from build123d import *

# Parameters (mm, degrees)
BOSS_EXTRUDE1_DEPTH = 25.4
SKETCH2_R           = 6
SKETCH2_R_2         = 5
CUT_EXTRUDE1_DEPTH  = 26.4
FILLET1_R           = 5


with BuildPart() as part:
    # Sketch1 → Boss-Extrude1 (new body)
    with BuildSketch(Plane(origin=(0, 0, 0), x_dir=(0, 0, -1), z_dir=(1, 0, 0))):
        with BuildLine():
            Line((12.7, 0), (12.7, -12.7))
            Line((12.7, -12.7), (38.1, -12.7))
            Line((38.1, -12.7), (38.1, -25.5))
            Line((38.1, -25.5), (-38.1, -25.5))
            Line((-38.1, -25.5), (-38.1, -12.7))
            Line((-38.1, -12.7), (-38.1, 0))
            Line((-38.1, 0), (-12.7, 0))
            ThreePointArc((-12.7, 0), (0, 12.7), (12.7, 0))
        make_face()
    extrude(amount=BOSS_EXTRUDE1_DEPTH)

    # Sketch2 → Cut-Extrude1 (cut, through all)
    with BuildSketch(Plane(origin=(25.4, 0, 0), x_dir=(0, 0, -1), z_dir=(1, 0, 0))):
        Circle(SKETCH2_R)
        with Locations((-25.2, -7.7)):
            Circle(SKETCH2_R_2)
    extrude(amount=-CUT_EXTRUDE1_DEPTH, mode=Mode.SUBTRACT)

    # Fillet1
    fillet1_edges = [part.edges().sort_by_distance(p)[0] for p in [
        (12.7, 0, 38.1),
    ]]
    fillet(fillet1_edges, radius=FILLET1_R)


solid = part.part
Source: CAD feature listing. Evaluate the final solid. Frame: model axes, mm. A direction names the side the tool comes from. Round coordinates to 2 decimals unless told otherwise and drop trailing zeros. Loops run counter-clockwise (first coordinate to the right, second up) from the corner with the lowest first, then second, coordinate; pieces in that order, holes last.
Q1. Mould query, pull axis Y, two halves, no side actions, for faces 4 (the face through (13, -25.5, -1)), 5 (the face through (13, 0, 6)), 6 (the face through (13, -19, -38.1)). Classes: pulls with the +Y half, pulls with the -Y half, needs draft (parallel to the pull), parting line crosses it, or undercut.
Q2. Section D-D, the plane y = 7.5. Return loops of the section in (x, z).
Q3. Section B-B, the plane y = -7.7. Return loops of the section in (x, z).
Q4. Ray query, line 1 (Y direction, x = 16.75, z = 0); line 2 (Y direction, x = 3.25, z = -14); line 3 (Z direction, x = 15.5, y = -5.5). Return the intervals inside material, ascending.
Q5. Section A-A, the plane z = 0. Return loops of the section in (x, y), plus the area to 3 significant figures.
Q6. First-contact query: P1, Ø6, axis at x = 8.5, z = 22, coming from the +Y side; P2, Ø1, axis at x = 19, z = 9, coming from the +Y side; P3, Ø10, axis at x = 15, y = -4, coming from the -Z side. Flat tips, straight axial feed; report the tip coordinate or a pass-through.
Q7. Access query for faces 1 (the face through (13, -12.7, -25)), 2 (the face through (13, 0, 23)), 3 (the face through (13, -15, 38.1)). Directions: +Z, -Z, +X, -X, +Y, -Y. A direction counts if a zero-diameter tool reaches every point of the face in a straight line with its end or side. Return the directions, or none.
Q8. Section C-C, the plane x = 17.5. Return loops of the section in (y, z).
Solutions:
1. face 4: pulls with the -Y half
1. face 5: undercut
1. face 6: needs draft
2. outline: (0, -10.25) - (25.4, -10.25) - (25.4, 10.25) - (0, 10.25) - close
3. outline: (0, -12.7) - (25.4, -12.7) - (25.4, 20.2) - (0, 20.2) - close; (0, 30.2) - (25.4, 30.2) - (25.4, 38.1) - (0, 38.1) - close
4. line 1: y = -25.5 to -6, 6 to 12.7
4. line 2: y = -25.5 to -12.7
4. line 3: z = -12.7 to -2.4, 2.4 to 20.71, 29.69 to 38.1
5. outline: (0, -25.5) - (25.4, -25.5) - (25.4, -6) - (0, -6) - close; (0, 6) - (25.4, 6) - (25.4, 12.7) - (0, 12.7) - close
5. area: 665 mm2
6. P1: stops at y = 0
6. P2: stops at y = 9.44
6. P3: stops at z = -12.7
7. face 1: -Z, +X, -X, +Y
7. face 2: +Z, +X, -X, +Y
7. face 3: +Z, +X, -X, +Y, -Y
8. outline: (-25.5, -38.1) - (-12.7, -38.1) - (-12.7, -12.7) - (0, -12.7) arc R12.7 ccw to (0, 12.7) - (0, 33.1) arc R5 ccw to (-5, 38.1) - (-25.5, 38.1) - close; hole circle Ø10 at (-7.7, 25.2); hole circle Ø12 at (0, 0)
